```python
from build123d import *

# Parameters (mm, degrees)
SKETCH1_R                = 50
BOSS_EXTRUDE1_DEPTH      = 27
BOSS_EXTRUDE2_REACH      = 141.133
BOSS_EXTRUDE2_END_RADIUS = 50
SKETCH2_R                = 32.5
SKETCH3_R                = 26.25
BOSS_EXTRUDE3_DEPTH      = 5
BODY_MOVE_COPY2_ANGLE    = 120


with BuildPart() as part:
    # Sketch1 → Boss-Extrude1 (new, symmetric)
    with BuildSketch(Plane.XY):
        Circle(SKETCH1_R)
    extrude(amount=BOSS_EXTRUDE1_DEPTH, both=True)

    # Boss-Extrude2: up to this cylinder (the profile starts outside it)
    boss_extrude2_end = Plane(origin=(0, 0, 0), z_dir=(0, 0, -1)) * Cylinder(BOSS_EXTRUDE2_END_RADIUS, 383.266, mode=Mode.PRIVATE)
    # Sketch2 → Boss-Extrude2 (add, up to the surface)
    with BuildSketch(Plane(origin=(77, 0, 0), x_dir=(0, 0, -1), z_dir=(1, 0, 0)), mode=Mode.PRIVATE) as boss_extrude2_sk1:
        Circle(SKETCH2_R)
    boss_extrude2_tool1 = extrude(boss_extrude2_sk1.sketch, amount=-BOSS_EXTRUDE2_REACH, mode=Mode.PRIVATE) - boss_extrude2_end
    add(boss_extrude2_tool1.solids().sort_by_distance((77, 0, 0))[0])

    # Sketch3 → Boss-Extrude3 (add)
    with BuildSketch(Plane(origin=(77, 0, 0), x_dir=(0, 0, -1), z_dir=(1, 0, 0))):
        Circle(SKETCH3_R)
    extrude(amount=BOSS_EXTRUDE3_DEPTH)


with BuildPart() as part_1:
    # Body-Move/Copy1: moved
    add(part.part.moved(Location((-82, 0, 0))))


with BuildPart() as part_2:
    # Body-Move/Copy2: moved
    add(part_1.part.rotate(Axis((0, 0, 0), (-0.5773502691896272, -0.5773502691896252, -0.5773502691896252)), BODY_MOVE_COPY2_ANGLE))


solid = part_2.part
```
The model under review builds one solid part; all positions refer to its coordinate system, in mm. A direction names the side the tool comes from. Round coordinates to 2 decimals unless told otherwise and drop trailing zeros. Loops run counter-clockwise (first coordinate to the right, second up) from the corner with the lowest first, then second, coordinate; pieces in that order, holes last. Notation, with made-up numbers: (13.25, 7) - (24.25, 7) arc R7 ccw to (24.25, 16) - close; hole circle Ø9 at (84.5, -0.5). An arc over 180 degrees is marked (long way). Use a Markdown table: item, result. Add a question column.
Q1. Add section A-A (y = 0). State the section outline as (x, z) points, plus the area to 3 significant figures.
Q2. For probe 1 along Y at (x, z) = (-12, -41); probe 2 along Z at (x, y) = (1, 6.5); probe 3 along X at (y, z) = (-27, -13), list the stretches that pass through material, from the lowest coordinate up.
Q3. Insertion check: pin 1 Ø4 at (y, z) = (9, -37.5) entering from +X; pin 2 Ø2 at (x, z) = (-10, -36.5) entering from -Y; pin 3 Ø3 at (y, z) = (23, -50.5) entering from +X. Each pin has a flat end and moves straight along its axis. Give the tip position at first contact, or say it passes through.
Q4. Add section C-C (z = -25). State the section outline as (x, y) points.
Q5. The part is to be moulded in two halves that separate along X. For faces 4 (the face through (15, 22, -5)), 5 (the face through (-12.45, -30.02, -19.9)), 6 (the face through (0, 29, -32)), say which applies: pulls with the +X half, pulls with the -X half, needs draft (parallel to the pull), parting line crosses it, or undercut.
Q6. Machinability: for faces 1 (the face through (-10.05, -24.25, -2.53)), 2 (the face through (0, -29, -32)), 3 (the face through (0, 0, 0)), which of the approach directions +Z, -Z, +X, -X, +Y, -Y give a long, thin tool a straight path to every point of the face, cutting with its end or side? Answer none if there is none.
Q7. Add section B-B (x = 0). State the section outline as (y, z) points.
Q8. Add section D-D (y = -7.5). State the section outline as (x, z) points.
Worked answers:
| question | item | result |
|---|---|---|
| 1 | outline | (-32.5, -44) arc R50 ccw (long way) to (32.5, -44) - (32.5, -5) - (26.25, -5) - (26.25, 0) - (-26.25, 0) - (-26.25, -5) - (-32.5, -5) - close |
| 1 | area | 10,100 mm² |
| 2 | probe 1 | -27 to 27 |
| 2 | probe 2 | -131.99 to 0 |
| 2 | probe 3 | -18.09 to 18.09 |
| 3 | pin 1 | x = 31.74 |
| 3 | pin 2 | y = -27 |
| 3 | pin 3 | x = 40 |
| 4 | outline | circle Ø65 at (0, 0) |
| 5 | face 4 | needs draft |
| 5 | face 5 | parting line crosses it |
| 5 | face 6 | undercut |
| 6 | face 1 | +Z |
| 6 | face 2 | -Z, -Y |
| 6 | face 3 | +Z, +X, -X, +Y, -Y |
| 7 | outline | (-32.5, -32) - (-27, -32) - (-27, -132) - (27, -132) - (27, -32) - (32.5, -32) - (32.5, -5) - (26.25, -5) - (26.25, 0) - (-26.25, 0) - (-26.25, -5) - (-32.5, -5) - close |
| 8 | outline | (-31.62, -43.27) arc R50 ccw (long way) to (31.62, -43.27) - (31.62, -5) - (25.16, -5) - (25.16, 0) - (-25.16, 0) - (-25.16, -5) - (-31.62, -5) - close |
